Build history of the part. All positions in model axes, mm. A direction names the side the tool comes from. Round coordinates to 2 decimals unless told otherwise and drop trailing zeros. Order: outer loops, then holes, each group sorted by start corner. A loop starts at its lowest first (then second) coordinate and runs counter-clockwise, first axis right, second up. Notation, with made-up numbers: (-35, 65.5) -> (-1, 65.5) arc R16 ccw to (-1, 90.5) -> close; hole circle Ø8 at (0.25, -27.75). An arc over 180 degrees is marked (long way). Answer as a JSON object with one key per item and string values.
from build123d import *

# Parameters (mm, degrees)
F0_R     = 35
F1_DEPTH = 100
F1_TAPER = -8
F2_T     = -5
F3_R     = 2


with BuildPart() as f1:
    # F0 (on Top) → F1 (new body)
    with BuildSketch(Plane.XY):
        Circle(F0_R)
    extrude(amount=F1_DEPTH, taper=F1_TAPER)

    # F2
    f2_openings = [f1.faces().sort_by_distance(p)[0] for p in [
        (0, 0, 100),
    ]]
    offset(amount=F2_T, openings=f2_openings, kind=Kind.INTERSECTION)

    # F3
    f3_edges = [f1.edges().sort_by_distance(p)[0] for p in [
        (-49.054083, 0, 100),
        (-44.004946, 0, 100),
        (-35, 0, 0),
    ]]
    fillet(f3_edges, radius=F3_R)


solid = f1.part
1) Cut at B-B, the plane z = 47.5. Give the cut face in (x, y), plus the area to 3 significant figures.
Checked values:
{"outline": "circle Ø83.35 at (0, 0); hole circle Ø73.25 at (0, 0)", "area": "1,240 mm²"}
2) Pull direction X, two halves, no side cores. Call faces 1 (the face through (-8.09, -36.41, 52.29)), 2 (the face through (0, 0, 0)), 3 (the face through (21.82, 34.22, 39.73)): pulls with the +X half, pulls with the -X half, needs draft (parallel to the pull), parting line crosses it, or undercut.
Checked values:
{"face 1": "undercut", "face 2": "needs draft", "face 3": "parting line crosses it"}
3) Flat gauge pins, fed straight in: pin 1 Ø1 at (y, z) = (22, 81) entering from -X; pin 2 Ø8 at (x, z) = (8.5, 14) entering from -Y; pin 3 Ø8 at (x, z) = (-14, 62.5) entering from +Y. Where does each tip first touch, or does it go through?
Checked values:
{"pin 1": "stops at x = -41.11", "pin 2": "stops at y = -36.93", "pin 3": "stops at y = 42.79"}
4) Probe L1, parallel to Z at x = 1, y = -8; L2, parallel to X at y = 21, z = 92.5; L3, parallel to Y at x = 34, z = 84.5. List the from-to ranges inside material, lowest first. Write a range as from..to.
Checked values:
{"L1": "z = 0..5", "L2": "x = -43.16..-37.47, 37.47..43.16", "L3": "y = -32.27..-24.36, 24.36..32.27"}
5) Cut at C-C, the plane z = 24. Give the cut face in (x, y), plus the area to 3 significant figures.
Checked values:
{"outline": "circle Ø76.75 at (0, 0); hole circle Ø66.65 at (0, 0)", "area": "1,140 mm²"}
6) Which spindle directions (+Z, -Z, +X, -X, +Y, -Y) get a long thin tool onto all of the face, cutting with end or side? Do faces 4 (the face through (0, 0, 5)), 5 (the face through (31, -34, 100)). Say none if no direction does.
Checked values:
{"face 4": "+Z", "face 5": "+Z, +X, -X, +Y, -Y"}
7) Cut at A-A, the plane x = 0. Give the cut face in (y, z).
Checked values:
{"outline": "(-48.73, 97.72) -> (-35.24, 1.72) arc R2 ccw to (-33.26, 0) -> (33.26, 0) arc R2 ccw to (35.24, 1.72) -> (48.73, 97.72) arc R2 ccw to (46.75, 100) -> (45.74, 100) arc R2 ccw to (43.76, 98.28) -> (30.65, 5) -> (-30.65, 5) -> (-43.76, 98.28) arc R2 ccw to (-45.74, 100) -> (-46.75, 100) arc R2 ccw to start"}
